Verification items for the finished model (mm, model axes). A direction names the side the tool comes from. Round coordinates to 2 decimals unless told otherwise and drop trailing zeros. Write each loop counter-clockwise with the first axis right and the second up, starting at its lowest first coordinate (ties: lowest second). Pieces come first, ordered by that corner, then holes. Notation, with made-up numbers: (72, 4) - (80, 4) arc R15 ccw to (80, 8) - close; hole circle Ø7 at (57.25, -10). An arc over 180 degrees is marked (long way). Answer as a JSON object with one key per item and string values. Group by question number.
1) Section check D-D (x = 78). Enter the section's corners in (y, z), then the cut area to 3 significant figures.
2) Set-up check for faces 1 (the cylindrical face through (85.68, -10.54, 7.56)), 2 (the cylindrical face through (62.31, -10.14, 9.04)): record each of +Z, -Z, +X, -X, +Y, -Y from which the full face is reachable in a straight line by a thin tool's end or side.
3) Section check A-A (z = 10). Enter the section's corners in (x, y), then the cut area to 4 significant figures.
4) Thickness scan on line 1 (Z direction, x = 60, y = -17); line 2 (X direction, y = -7, z = 8.5); line 3 (X direction, y = -18.75, z = 9.25). Record the ranges inside material, lowest first.
5) Section check C-C (y = -10). Enter the section's corners in (x, z).
6) Section check B-B (x = 10). Enter the section's corners in (y, z).
7) Mould release check, pull along Y, two halves, no side actions. Record for faces 3 (the flat face through (48, 0, 10)), 4 (the flat face through (73, -10, 10)), 5 (the flat face through (48, -10, 0)), 6 (the flat face through (48, -20, 10)): +Y half, -Y half, draft (parallel to the pull), parting line (faces both ways), or undercut.
8) Go/stop test with a flat-tipped pin: pin 1 Ø3 at (x, z) = (10, 10) entering from +Y. Record where the tip stops, or that it passes through.
```python
from build123d import *

# Parameters (mm, degrees)
F0_W     = 98
F0_H     = 20
F1_DEPTH = 20
F2_R     = 2.5
F3_DEPTH = 25
F4_R     = 2.5
F5_DEPTH = 20.001


with BuildPart() as f1:
    # F0 (on Front) → F1 (new body)
    with BuildSketch(Plane.XZ):
        with Locations((49, 10)):
            Rectangle(F0_W, F0_H)
    extrude(amount=F1_DEPTH)

    # F2 (on face) → F3 (cut)
    with BuildSketch(Plane.YZ.offset(98)):
        with Locations((-10, 10)):
            Circle(F2_R)
    extrude(amount=-F3_DEPTH, mode=Mode.SUBTRACT)

    # F4 (on face) → F5 (cut, through all)
    with BuildSketch(Plane.XZ.offset(20)):
        with Locations((10, 10)):
            Circle(F4_R)
        with Locations((60, 10)):
            Circle(F4_R)
    extrude(amount=-F5_DEPTH, mode=Mode.SUBTRACT)


solid = f1.part
```
Returned:
{
 "1": {"outline": "(-20, 0) - (0, 0) - (0, 20) - (-20, 20) - close; hole circle Ø5 at (-10, 10)", "area": "380 mm2"},
 "2": {"face 1": "+X", "face 2": "+Y, -Y"},
 "3": {"outline": "(0, -20) - (7.5, -20) - (7.5, 0) - (0, 0) - close; (12.5, -20) - (57.5, -20) - (57.5, 0) - (12.5, 0) - close; (62.5, -20) - (98, -20) - (98, -12.5) - (73, -12.5) - (73, -7.5) - (98, -7.5) - (98, 0) - (62.5, 0) - close", "area": "1,635 mm2"},
 "4": {"line 1": "0 to 7.5, 12.5 to 20", "line 2": "0 to 8, 12 to 58, 62 to 98", "line 3": "0 to 7.62, 12.38 to 57.62, 62.38 to 98"},
 "5": {"outline": "(0, 0) - (98, 0) - (98, 7.5) - (73, 7.5) - (73, 12.5) - (98, 12.5) - (98, 20) - (0, 20) - close; hole circle Ø5 at (10, 10); hole circle Ø5 at (60, 10)"},
 "6": {"outline": "(-20, 0) - (0, 0) - (0, 7.5) - (-20, 7.5) - close; (-20, 12.5) - (0, 12.5) - (0, 20) - (-20, 20) - close"},
 "7": {"face 3": "+Y half", "face 4": "undercut", "face 5": "draft", "face 6": "-Y half"},
 "8": {"pin 1": "through"}
}
